Work out the finished part from the listing and answer in its coordinate system (mm). A direction names the side the tool comes from. Round coordinates to 2 decimals unless told otherwise and drop trailing zeros. Loops run counter-clockwise (first coordinate to the right, second up) from the corner with the lowest first, then second, coordinate; pieces in that order, holes last. Notation, with made-up numbers: (-26.75, 18) -> (14.25, 18) arc R22 cw to (14.25, 31) -> close; hole circle Ø9 at (24, 21). An arc over 180 degrees is marked (long way). Use CSV: the item, a comma, the result in double quotes. Start each with the question number.
Autodesk Inventor part; units mm, degrees
ref_plane "YZ Plane" through (0, 0, 0) normal (1, 0, 0) x (0, 1, 0)
ref_plane "XZ Plane" through (0, 0, 0) normal (0, 1, 0) x (-1, 0, 0)
ref_plane "XY Plane" through (0, 0, 0) normal (0, 0, 1) x (1, 0, 0)
sketch "Sketch1" plane through (0, 0, 0) normal (0, 0, 1) x (1, 0, 0)
  line L0 (0, 0) -> (20, 0)
  line L1 (20, 35) -> (20, 45)
  line L2 (20, 45) -> (0, 45)
  line L3 (0, 45) -> (0, 0)
  line L4 (20, 0) -> (25, 0)
  line L5 (25, 0) -> (25, 35)
  line L6 (20, 35) -> (20, 0)
  line L7 (25, 0) -> (37, 0)
  line L8 (37, 0) -> (37, 35)
  line L9 (37, 35) -> (25, 35)
  line L10 (25, 35) -> (25, 0)
  line L11 (20, 45) -> (25, 35)
  line L12 (37, 0) -> (53, 0)
  line L13 (53, 0) -> (53, 35)
  line L14 (37, 35) -> (37, 0)
  arc A0 (37, 35) -> (53, 35) centre (45, 35) ccw
  line L15 (53, 0) -> (75, 0)
  line L16 (75, 0) -> (75, 20)
  line L17 (60, 35) -> (53, 35)
  line L18 (53, 35) -> (53, 0)
  arc A1 (75, 20) -> (60, 35) centre (60, 20) ccw
  arc A2 (53, 33.2665) -> (52.7831, 33.1498) centre (60, 20) ccw
  line L19 (75, 0) -> (78, 0)
  line L20 (78, 0) -> (78, 15)
  line L21 (78, 15) -> (75, 15)
  line L22 (75, 15) -> (75, 0)
  line L23 (78, 0) -> (105, 0)
  line L24 (105, 0) -> (105, 20)
  line L25 (105, 20) -> (78, 20)
  line L26 (78, 20) -> (78, 0)
  line L27 (105, 0) -> (108, 0)
  line L28 (108, 0) -> (108, 7.5)
  line L29 (108, 7.5) -> (105, 7.5)
  line L30 (105, 7.5) -> (105, 0)
  line L31 (108, 0) -> (130, 0)
  line L32 (130, 0) -> (130, 10)
  line L33 (130, 10) -> (108, 10)
  line L34 (108, 10) -> (108, 0)
  line L35 (164.0679, 0) -> (-30.9325, 0)
  line L36 (-30.9325, 35) -> (60, 35)
  line L37 (75, 35) -> (164.0679, 35)
  line L38 (60, 35) -> (75, 35)
  point P0 (53, 33.2665)
  dimension "d0" = 20
  dimension "d4" = 12
  dimension "d5" = 35
  dimension "d7" = 16
  dimension "d9" = 22
  dimension "d12" = 3
  dimension "d13" = 15
  dimension "d14" = 27
  dimension "d15" = 20
  dimension "d16" = 3
  dimension "d17" = 7.5
  dimension "d18" = 22
  dimension "d19" = 10
  dimension "d20" = 45
  dimension "d21" = 5
  dimension "d22" = 15
  dimension "d23" = 7
revolve "Revolution1" add sketch "Sketch1" angle 360 about axis through (164.0679, 0, 0) along (-1, 0, 0) contours L3 L36 L6 L0 | L6 L36 L5 L4 | L3 L2 L1 L36 | L5 L9 L8 L7 | L1 L11 L36 | L8 A0 A2 L13 L12 | L13 L17 A1 L16 L15 | L16 L21 L20 L19 | L20 L26 L25 L24 L23 | L24 L29 L28 L27 | L28 L34 L33 L32 L31
chamfer "Chamfer1" distance 2 angle 45 1 edges at (105, -20, 0)
chamfer "Chamfer2" distance 2 angle 45 1 edges at (130, -10, 0)
thread "Thread1"
thread "Thread2"
properties part number "Tarefa 2" material "Bronze, Cast"
Q1. Section A-A, the plane x = 81.5 is taken. Write down the section's boundary in (y, z), and give its area (3 significant figures).
Q2. For a pull along X with two mould halves and no side action, classify faces 1 (the flat face through (78, 3, -15)), 2 (the cylindrical face through (117.86, -2.17, 9.76)), 3 (the conical face through (104.875, -2.36, -17.971)) as pulls with the +X half, pulls with the -X half, needs draft (parallel to the pull), parting line crosses it, or undercut.
Q3. Which of the six approach directions +Z, -Z, +X, -X, +Y, -Y give full straight-line access (tool end or side, diameter ignored) to faces 4 (the cylindrical face through (90.325, -4.336, 19.524)), 5 (the flat face through (75, 3, -15)), 6 (the flat face through (130, 0, 0))?
Q4. Each of these flat-tipped pins is pushed along its axis until it touches: pin 1 (1 mm diameter, centred on x = 59, y = -4.5, fed in from +Z); pin 2 (1 mm diameter, centred on y = 25, z = -31, fed in from +X); pin 3 (5 mm diameter, centred on x = 103, y = -6.5, fed in from +Z). Where does it stop, or does it pass through?
Q5. Section B-B, the plane x = 23 is taken. Write down the section's boundary in (y, z), and give its area (3 significant figures).
Q6. Straight lines are drawn through the part: line 1 (X direction, y = 24.5, z = 15); line 2 (X direction, y = 40, z = 13); line 3 (Z direction, x = 67.5, y = -27). For each, find the intervals that lie inside material, in ascending order. Write a range as from..to.
Report:
1,outline,"circle Ø40 at (0, 0)"
1,area,"1,260 mm²"
2,face 1,"undercut"
2,face 2,"needs draft"
2,face 3,"pulls with the +X half"
3,face 4,"+X"
3,face 5,"none"
3,face 6,"+Z, -Z, +X, +Y, -Y"
4,pin 1,"stops at z = 34.77"
4,pin 2,"stops at x = 22.84"
4,pin 3,"stops at z = 19.6"
5,outline,"circle Ø78 at (0, 0)"
5,area,"4,780 mm²"
6,line 1,"x = 0..40.03, 49.97..72.2"
6,line 2,"x = 0..21.47"
6,line 3,"z = -18.96..18.96"
